Check sheet for the modelled part. Datum: model origin and axes. Units: mm. Face numbers are marked on the shaded views. A direction names the side the tool comes from. Round coordinates to 2 decimals unless told otherwise and drop trailing zeros. Write each loop counter-clockwise with the first axis right and the second up, starting at its lowest first coordinate (ties: lowest second). Pieces come first, ordered by that corner, then holes. Notation, with made-up numbers: (63, -31.5) -> (121, -31.5) arc R5 cw to (121, -24.5) -> close; hole circle Ø5 at (-9.75, 0). An arc over 180 degrees is marked (long way). One line per item, written item: value.
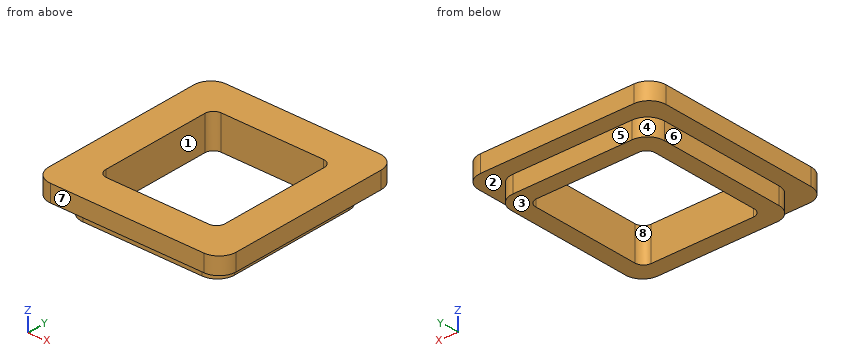
Autodesk Fusion 360 part; units mm, degrees
sketch "Esboço1" plane through (0, 0, 0) normal (0, 0, 1) x (1, 0, 0)
  line L0 (9, 9.5) -> (-9, 9.5)
  line L1 (-9, 9.5) -> (-9, -9.5)
  line L2 (-9, -9.5) -> (9, -9.5)
  line L3 (9, -9.5) -> (9, 9.5)
  line L4 (9, 9.5) -> (-9, -9.5) construction
  line L5 (-9, 9.5) -> (9, -9.5) construction
  line L6 (-7, -7.5) -> (7, -7.5)
  line L7 (7, -7.5) -> (7, 7.5)
  line L8 (7, 7.5) -> (-7, 7.5)
  line L9 (-7, 7.5) -> (-7, -7.5)
  dimension "d1" = 18
  dimension "d2" = 19
  dimension "d3" = -2
extrude "Extrusão1" add sketch "Esboço1" along normal blind 2
sketch "Esboço2" plane through (0, 0, 2) normal (0, 0, 1) x (-1, 0, 0)
  line L0 (7, 7.5) -> (7, -7.5)
  line L1 (7, -7.5) -> (-7, -7.5)
  line L2 (-7, -7.5) -> (-7, 7.5)
  line L3 (-7, 7.5) -> (7, 7.5)
  line L4 (-9, 9.5) -> (-9, -9.5)
  line L5 (-9, -9.5) -> (9, -9.5)
  line L6 (9, -9.5) -> (9, 9.5)
  line L7 (9, 9.5) -> (-9, 9.5)
  line L8 (-11, 9.5) -> (-11, -9.5)
  line L9 (-9, -11.5) -> (9, -11.5)
  line L10 (11, -9.5) -> (11, 9.5)
  line L11 (9, 11.5) -> (-9, 11.5)
  arc A0 (11, 9.5) -> (9, 11.5) centre (9, 9.5) ccw
  arc A1 (-9, 11.5) -> (-11, 9.5) centre (-9, 9.5) ccw
  arc A2 (-11, -9.5) -> (-9, -11.5) centre (-9, -9.5) ccw
  arc A3 (9, -11.5) -> (11, -9.5) centre (9, -9.5) ccw
  dimension "d7" = 2
extrude "Extrusão2" add sketch "Esboço2" along normal blind 2 contours L4 L5 L6 L7 | L8 L9 L10 L11 A0 A1 A2 A3
fillet "Arredondamento1" radius 2 4 edges at (-9, 9.5, 1) (-9, -9.5, 1) (9, 9.5, 1) (9, -9.5, 1)
fillet "Arredondamento2" radius 1 4 edges at (-7, 7.5, 2) (-7, -7.5, 2) (7, -7.5, 2) (7, 7.5, 2)
Item 1: Sectioned sample at C-C (z = 3.55). Enter the section's corners in (x, y), then the cut area to 3 significant figures.
Result set:
outline: (-11, -9.5) arc R2 ccw to (-9, -11.5) -> (9, -11.5) arc R2 ccw to (11, -9.5) -> (11, 9.5) arc R2 ccw to (9, 11.5) -> (-9, 11.5) arc R2 ccw to (-11, 9.5) -> close; hole (-7, -6.5) arc R1 ccw to (-6, -7.5) -> (6, -7.5) arc R1 ccw to (7, -6.5) -> (7, 6.5) arc R1 ccw to (6, 7.5) -> (-6, 7.5) arc R1 ccw to (-7, 6.5) -> close
area: 293 mm^2
Item 2: Sectioned sample at B-B (y = -5.25). Enter the section's corners in (x, z).
Result set:
outline: (-11, 2) -> (-9, 2) -> (-9, 0) -> (-7, 0) -> (-7, 4) -> (-11, 4) -> close; (7, 0) -> (9, 0) -> (9, 2) -> (11, 2) -> (11, 4) -> (7, 4) -> close
Item 3: Sectioned sample at D-D (y = -8.5). Enter the section's corners in (x, z), then the cut area to 3 significant figures.
Result set:
outline: (-11, 2) -> (-8.73, 2) -> (-8.73, 0) -> (8.73, 0) -> (8.73, 2) -> (11, 2) -> (11, 4) -> (-11, 4) -> close
area: 78.9 mm^2
Item 4: Sectioned sample at A-A (x = 4.25). Enter the section's corners in (y, z).
Result set:
outline: (-11.5, 2) -> (-9.5, 2) -> (-9.5, 0) -> (-7.5, 0) -> (-7.5, 4) -> (-11.5, 4) -> close; (7.5, 0) -> (9.5, 0) -> (9.5, 2) -> (11.5, 2) -> (11.5, 4) -> (7.5, 4) -> close
Item 5: Release check for a two-part mould opening along X. For the marked faces 6, 7 and 8 record: pulls with the +X half, pulls with the -X half, needs draft (parallel to the pull), parting line crosses it, or undercut.
Result set:
face 6: pulls with the -X half
face 7: needs draft
face 8: undercut
Item 6: Material ranges on line 1 along X through (y, z) = (1, 0.25); line 2 along Y through (x, z) = (1, 2.4); line 3 along X through (y, z) = (2, 2.1), recorded low to high.
Result set:
line 1: -9 to -7, 7 to 9
line 2: -11.5 to -7.5, 7.5 to 11.5
line 3: -11 to -7, 7 to 11
Item 7: Tool access check on the marked faces 1, 2, 3, 4 and 5. Record the directions out of +Z, -Z, +X, -X, +Y, -Y that give a thin tool (end or side, any length) a straight path to the whole face; none if there is none.
Result set:
face 1: +Z, -Z
face 2: -Z
face 3: -Z, +X, -X, +Y, -Y
face 4: -Z, -X, +Y
face 5: -Z, +X, -X, +Y
Item 8: Depth check by flat-ended pin: pin 1 (1.6 mm diameter, centred on x = 2.5, z = 0.5, fed in from -Y); pin 2 (1.6 mm diameter, centred on y = -1.5, z = 0.5, fed in from -X); pin 3 (1 mm diameter, centred on y = 2.5, z = 0.5, fed in from +X). Enter the tip coordinate at first touch or a pass-through.
Result set:
pin 1: y = -9.5
pin 2: x = -9
pin 3: x = 9
